from build123d import *

# Parameters (mm, degrees)
SKIZZE1_R                       = 49.571868138
AUFSATZ_LINEAR_AUSTRAGEN6_DEPTH = 33
LINEAR_AUSTRAGEN_D_NN9_DEPTH    = 33


with BuildPart() as part:
    # Skizze1 → Aufsatz-Linear austragen6 (new body)
    with BuildSketch(Plane(origin=(0, 0, 0), x_dir=(1, 0, 0), z_dir=(0, 1, 0))):
        with Locations(Location((0, 0, 0), (0, 0, 270))):
            Circle(SKIZZE1_R)
    extrude(amount=AUFSATZ_LINEAR_AUSTRAGEN6_DEPTH)

    # Skizze2 → Linear-Austragen-Dünn9 (add)
    with BuildSketch(Plane(origin=(0, 33, 0), x_dir=(1, 0, 0), z_dir=(0, 1, 0))):
        Polygon((-8.848811268, 0), (-30.694314085, 0), (-30.694314085, 26.615565141), (0, 26.615565141), (0, 10.300569366), (80, 10.300569366), (80, 106.615565141), (-110.694314085, 106.615565141), (-110.694314085, -80), (-8.848811268, -80), align=None)
        Polygon((0, 10.024044014), (27.099484508, 10.024044014), (27.099484508, -17.490228521), (-8.987073944, -17.490228521), (-8.987073944, 0), (-88.987073944, 0), (-88.987073944, -97.490228521), (107.099484508, -97.490228521), (107.099484508, 90.024044014), (0, 90.024044014), align=None)
    extrude(amount=LINEAR_AUSTRAGEN_D_NN9_DEPTH)


solid = part.part
Part model, mm, in its own coordinate system. A direction names the side the tool comes from. Give positions to 0.01 mm unless a question says otherwise; leave off trailing zeros. Order: outer loops, then holes, each group sorted by start corner. A loop starts at its lowest first (then second) coordinate and runs counter-clockwise, first axis right, second up. Notation, with made-up numbers: (64, 61) - (91, 61) arc R28 ccw to (91, 82) - close; hole circle Ø9 at (-15, 27). An arc over 180 degrees is marked (long way). Use a Markdown table: item, result.
1) 3-axis set-ups, long thin cutter, end or side, ignore diameter. For faces 1 (the flat face through (-88.987, 49, 89)), 2 (the flat face through (94, 49, -90.024)), 3 (the flat face through (107.099, 49, 5)), 4 (the flat face through (-8.849, 49, 9)), 5 (the flat face through (-3, 33, -51)): which of +Z, -Z, +X, -X, +Y, -Y reach the whole face in a straight line?
Checked values:
| item | result |
|---|---|
| face 1 | +Z, -X, +Y, -Y |
| face 2 | -Z, +X, +Y, -Y |
| face 3 | +Z, -Z, +X, +Y, -Y |
| face 4 | +Y |
| face 5 | -Y |
2) Saw through at B-B on x = -3. List the corners of the cut face in (y, z).
Checked values:
| item | result |
|---|---|
| outline | (0, -49.48) - (33, -49.48) - (33, -106.62) - (66, -106.62) - (66, -26.62) - (33, -26.62) - (33, 17.49) - (66, 17.49) - (66, 97.49) - (33, 97.49) - (33, 49.48) - (0, 49.48) - close |
3) Saw through at A-A on y = 41. List the corners of the cut face in (x, z).
Checked values:
| item | result |
|---|---|
| outline | (-110.69, -106.62) - (80, -106.62) - (80, -90.02) - (107.1, -90.02) - (107.1, 97.49) - (-88.99, 97.49) - (-88.99, 80) - (-110.69, 80) - close; hole (-30.69, -26.62) - (0, -26.62) - (0, -10.02) - (27.1, -10.02) - (27.1, 17.49) - (-8.85, 17.49) - (-8.85, 0) - (-30.69, 0) - close |
4) Saw through at C-C on z = 22. List the corners of the cut face in (x, y).
Checked values:
| item | result |
|---|---|
| outline | (-110.69, 33) - (-44.42, 33) - (-44.42, 0) - (44.42, 0) - (44.42, 33) - (107.1, 33) - (107.1, 66) - (-110.69, 66) - close |
5) Two-plate mould, pull along Z, no slides. Class faces 6 (the flat face through (-100, 49, 80)), 7 (the flat face through (-20, 49, 0)), 8 (the flat face through (80, 49, -98)): +Z half, -Z half, draft (parallel to the pull), parting line (faces both ways), or undercut.
Checked values:
| item | result |
|---|---|
| face 6 | +Z half |
| face 7 | undercut |
| face 8 | draft |
6) Probe L1, parallel to Z at x = 9, y = 57; L2, parallel to X at y = 57, z = -8.5; L3, parallel to Y at x = -45.5, z = -23. List the from-to ranges inside material, lowest first. Write a range as from..to.
Checked values:
| item | result |
|---|---|
| L1 | -106.62..-10.02, 17.49..97.49 |
| L2 | -110.69..-30.69, 27.1..107.1 |
| L3 | 33..66 |
7) Saw through at D-D on y = 9.5. List the corners of the cut face in (x, z), plus the area to 3 significant figures.
Checked values:
| item | result |
|---|---|
| outline | circle Ø99.14 at (0, 0) |
| area | 7,720 mm² |
8) Flat gauge pins, fed straight in: P1, Ø22, axis at x = -11.5, z = -15, coming from the +Y side; P2, Ø5, axis at y = 50.5, z = -99.5, coming from the +X side; P3, Ø8, axis at x = 100, y = 57, coming from the -Z side. Where does each tip first touch, or does it go through?
Checked values:
| item | result |
|---|---|
| P1 | y = 33 |
| P2 | x = 80 |
| P3 | z = -90.02 |
